from build123d import *

# Parameters (mm, degrees)
BOSS_EXTRUDE2_DEPTH      = 10
BOSS_EXTRUDE2_DEPTH_BACK = 10
SKETCH3_R                = 1.5
TOP_FORM_DEPTH           = 105.378363468
TOP_FORM_DEPTH_BACK      = 105.378363468
SKETCH12_OUTSIDE_W       = 129.881
SKETCH12_OUTSIDE_H       = 44.03


with BuildPart() as part:
    # Sketch3 → Boss-Extrude2 (new, two sides: drawn at the far end of the back side and taken through both)
    with BuildSketch(Plane.XY.offset(-BOSS_EXTRUDE2_DEPTH_BACK)):
        with BuildLine():
            Line((1.282575537, 3.523847328), (-41.906339045, 19.243326686))
            Line((-41.906339045, 19.243326686), (-82.109540341, 19.243326686))
            Line((-82.109540341, 19.243326686), (-99.100622615, 9.433520762))
            Line((-99.100622615, 9.433520762), (-102.100622615, 3))
            Line((-102.100622615, 3), (-100, 0))
            Line((-100, 0), (-83.2287914, 11.743326686))
            Line((-83.2287914, 11.743326686), (-43.2287914, 11.743326686))
            Line((-43.2287914, 11.743326686), (-1.282575537, -3.523847328))
            ThreePointArc((-1.282575537, -3.523847328), (3.523847328, -1.282575537), (1.282575537, 3.523847328))
        make_face()
        Circle(SKETCH3_R, mode=Mode.SUBTRACT)
    extrude(amount=BOSS_EXTRUDE2_DEPTH + BOSS_EXTRUDE2_DEPTH_BACK)

    # Sketch12 outside → top-form (cut, two sides: drawn at the far end of the back side and taken through both)
    # profile 1 of 2: a face of its own
    with BuildSketch(Plane(origin=(0, 0, 0), x_dir=(1, 0, 0), z_dir=(0, 1, 0)).offset(-TOP_FORM_DEPTH_BACK)):
        with Locations((-49.1755, 0)):
            Rectangle(SKETCH12_OUTSIDE_W, SKETCH12_OUTSIDE_H)
        Polygon((3.523847328, -3.75), (3.523847328, 3.75), (3.75, 10), (-3.75, 10), (-102.100622615, 7.5), (-102.100622615, -7.5), (-3.75, -10), (3.75, -10), align=None, mode=Mode.SUBTRACT)
    # profile 2 of 2: a face of its own
    with BuildSketch(Plane(origin=(0, 0, 0), x_dir=(1, 0, 0), z_dir=(0, 1, 0)).offset(-TOP_FORM_DEPTH_BACK)):
        with BuildLine():
            ThreePointArc((0.923847328, -1.6), (2.523847328, 0), (0.923847328, 1.6))
            Line((0.923847328, 1.6), (-1.076152672, 1.6))
            ThreePointArc((-1.076152672, 1.6), (-2.676152672, 0), (-1.076152672, -1.6))
            Line((-1.076152672, -1.6), (0.923847328, -1.6))
        make_face()
    extrude(amount=TOP_FORM_DEPTH + TOP_FORM_DEPTH_BACK, mode=Mode.SUBTRACT)

    # spikes cone 1 section (through the dimple's axis) → spikes (revolve)
    with BuildSketch(Plane(origin=(-98.771271934, 0.860364655, 6.08430449), x_dir=(0, 0, 1), z_dir=(0.819152044, 0.573576436, 0))):
        Polygon((0, 0), (0.75, 0), (0, 3.528472582), align=None)
    revolve(axis=Axis((-98.771271934, 0.860364655, 6.08430449), (0.573576436, -0.819152044, 0)))

    # spikes cone 2 section (through the dimple's axis) → spikes cone 2 (revolve)
    with BuildSketch(Plane(origin=(-98.771271934, 0.860364655, -6.08430449), x_dir=(0, 0, 1), z_dir=(0.819152044, 0.573576436, 0))):
        Polygon((0, 0), (0.75, 0), (0, 3.528472582), align=None)
    revolve(axis=Axis((-98.771271934, 0.860364655, -6.08430449), (0.573576436, -0.819152044, 0)))


solid = part.part
Model file for the job. Use its own axes, mm. A direction names the side the tool comes from. Round coordinates to 2 decimals unless told otherwise and drop trailing zeros. Order: outer loops, then holes, each group sorted by start corner. A loop starts at its lowest first (then second) coordinate and runs counter-clockwise, first axis right, second up. Notation, with made-up numbers: M 16,39.5 L 44,39.5 A26 cw 44,54.5 Z; hole C 36.5,-14 d1. An arc over 180 degrees is marked long. Write each question's results on one line, items separated by ' | '. Start each with the question number.
(1) Which spindle directions (+Z, -Z, +X, -X, +Y, -Y) get a long thin tool onto all of the face, cutting with end or side? Do faces 1 (the face through (-64, 11.743, 0)), 2 (the face through (2.523, -0.041, 0.035)), 3 (the face through (-2, 1, -10)), 4 (the face through (3.613, -0.018, 6.224)). Say none if no direction does.
(2) Probe probe 1 along Y at (x, z) = (0, 7); probe 2 along Y at (x, z) = (-46, -5.5); probe 3 along Y at (x, z) = (-86.5, -4.75). List the from-to ranges inside material, lowest first. Write a range as from..to.
(3) Saw through at D-D, the plane x = -32. Give the cut face in (y, z), then the cut area to 3 significant figures.
(4) Saw through at B-B, the plane x = 0. Give the cut face in (y, z), then the cut area to 3 significant figures.
(5) Two-plate mould, pull along Y, no slides. Class faces 5 (the face through (3.61, -0.02, -6.14)), 6 (the face through (-100.58, 6.26, -0.11)), 7 (the face through (-1.5, 0.07, -5.81)): pulls with the +Y half, pulls with the -Y half, needs draft (parallel to the pull), parting line crosses it, or undercut.
(6) Saw through at A-A, the plane z = 2.5. Give the cut face in (x, y).
(7) Saw through at C-C, the plane y = 14.5. Give the cut face in (x, z), then the cut area to 3 significant figures.
(8) Drop flat-ended pins along their axis: pin 1 (6 mm diameter, centred on y = 11.5, z = -6.5, fed in from -X); pin 2 (1.5 mm diameter, centred on x = -24, z = -7, fed in from +Y); pin 3 (1 mm diameter, centred on x = -15, z = -4.5, fed in from +Y). Give the stop position or say it passes through.
Established:
1) face 1: +Z, -Z, -Y | face 2: +Y, -Y | face 3: -Z, +X, -X, +Y, -Y | face 4: +X, +Y, -Y
2) probe 1: y = -3.75..-1.5, 1.5..3.99 | probe 2: y = 11.74..19.24 | probe 3: y = 9.45..16.71
3) outline: M 7.66,-9.28 L 15.64,-9.28 L 15.64,9.28 L 7.66,9.28 Z | area: 148 mm^2
4) outline: M -3.75,-10 L -1.5,-10 L -1.5,-1.6 L -3.75,-1.6 Z; M -3.75,1.6 L -1.5,1.6 L -1.5,10 L -3.75,10 Z; M 1.5,-10 L 3.99,-10 L 3.99,-1.6 L 1.5,-1.6 Z; M 1.5,1.6 L 3.99,1.6 L 3.99,10 L 1.5,10 Z | area: 79.6 mm^2
5) face 5: needs draft | face 6: pulls with the +Y half | face 7: undercut
6) outline: M -102.1,3 L -100,0 L -83.23,11.74 L -43.23,11.74 L -1.28,-3.52 A3.75 ccw 3.52,-1.28 L 3.52,1.28 A3.75 ccw 1.28,3.52 L -41.91,19.24 L -82.11,19.24 L -99.1,9.43 Z; hole C 0,0 d3
7) outline: M -90.33,-7.8 L -28.87,-9.36 L -28.87,9.36 L -90.33,7.8 Z | area: 1,050 mm^2
8) pin 1: stops at x = -99.54 | pin 2: stops at y = 13 | pin 3: stops at y = 9.63
